from build123d import *

# Parameters (mm, degrees)
SKETCH_1_R          = 17
EXTRUDE_1_DEPTH     = 2
EXTRUDE_2_DEPTH     = 1
FILLET_1_R          = 1.55
FILLET_2_R          = 0.8
SKETCH_3_R          = 7
CUT_EXTRUDE_1_DEPTH = 4
SKETCH_4_R          = 1.25
CUT_EXTRUDE_2_DEPTH = 4.0000001


with BuildPart() as part:
    # ｽｹｯﾁ1 → ﾎﾞｽ - 押し出し1 (new body)
    with BuildSketch(Plane.XY):
        Circle(SKETCH_1_R)
    extrude(amount=EXTRUDE_1_DEPTH)

    # ｽｹｯﾁ2 → ﾎﾞｽ - 押し出し2 (add)
    with BuildSketch(Plane.XY.offset(2)):
        with BuildLine():
            Line((-1.5, 14.422205102), (-1.5, 12.5))
            Line((-1.5, 12.5), (1.5, 12.5))
            Line((1.5, 12.5), (1.5, 14.422205102))
            ThreePointArc((1.5, 14.422205102), (0, 14.5), (-1.5, 14.422205102))
        make_face()
        with BuildLine():
            Line((1.5, 12.5), (-1.5, 12.5))
            Line((-1.5, 12.5), (-1.5, 14.422205102))
            ThreePointArc((-1.5, 14.422205102), (-9.708243919, -10.770329614), (14.5, 0))
            ThreePointArc((14.5, 0), (10.770329614, 9.708243919), (1.5, 14.422205102))
            Line((1.5, 14.422205102), (1.5, 12.5))
        make_face()
        with BuildLine():
            Line((-1.5, 16.5), (-1.5, 14.422205102))
            ThreePointArc((-1.5, 14.422205102), (0, 14.5), (1.5, 14.422205102))
            Line((1.5, 14.422205102), (1.5, 16.5))
            Line((1.5, 16.5), (-1.5, 16.5))
        make_face()
    extrude(amount=EXTRUDE_2_DEPTH)

    # ﾌｨﾚｯﾄ1
    fillet_1_edges = [part.edges().sort_by_distance(p)[0] for p in [
        (-1.5, 14.422205102, 2.5),
        (1.5, 14.422205102, 2.5),
    ]]
    fillet(fillet_1_edges, radius=FILLET_1_R)

    # ﾌｨﾚｯﾄ2
    fillet_2_edges = [part.edges().sort_by_distance(p)[0] for p in [
        (1.5, 16.5, 2.5),
        (-1.5, 16.5, 2.5),
    ]]
    fillet(fillet_2_edges, radius=FILLET_2_R)

    # ｽｹｯﾁ3 → ｶｯﾄ - 押し出し1 (cut, through all)
    with BuildSketch(Plane.XY.offset(3)):
        Circle(SKETCH_3_R)
    extrude(amount=-CUT_EXTRUDE_1_DEPTH, mode=Mode.SUBTRACT)

    # ｽｹｯﾁ4 → ｶｯﾄ - 押し出し2 (cut, through all)
    with BuildSketch(Plane(origin=(0, 0, 0), x_dir=(-1, 0, 0), z_dir=(0, 0, -1))):
        with Locations((0, 12)):
            Circle(SKETCH_4_R)
        with Locations((12, 0)):
            Circle(SKETCH_4_R)
        with Locations((0, -12)):
            Circle(SKETCH_4_R)
        with Locations((-12, 0)):
            Circle(SKETCH_4_R)
    extrude(amount=-CUT_EXTRUDE_2_DEPTH, mode=Mode.SUBTRACT)


solid = part.part
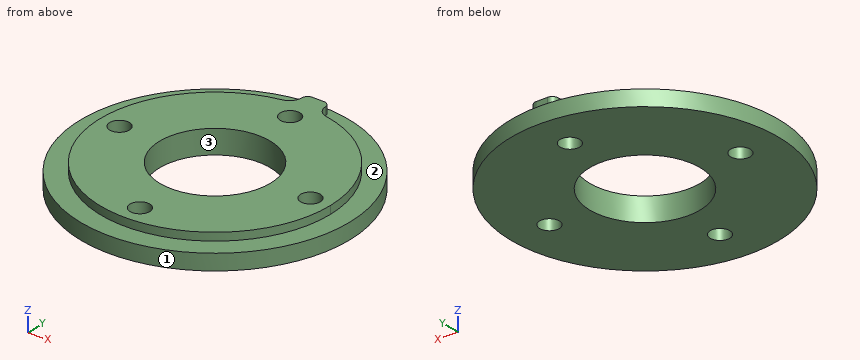
Input: part model. Units: mm. Frame: model coordinates. Face numbers are marked on the shaded views. Coordinates: 2 decimals unless noted, no trailing zeros. Loops run counter-clockwise (first coordinate to the right, second up) from the corner with the lowest first, then second, coordinate; pieces in that order, holes last.
Q1. Cut plane C-C (z = 0.65). Output: boundary loops of the cut face in (x, y), then the cut area to 3 significant figures.
Q2. Material intervals for line 1 (Y direction, x = 0, z = 1.5); line 2 (X direction, y = -1, z = 1.95); line 3 (Y direction, x = 11, z = 1.45), sorted ascending.
Q3. Draft query along Y for the marked faces 1, 2 and 3. Return one class per face: +Y half, -Y half, draft (parallel to the pull), parting line (faces both ways), or undercut.
Q4. Cut plane A-A (x = 0). Output: boundary loops of the cut face in (y, z).
Q5. Cut plane B-B (y = 12). Output: boundary loops of the cut face in (x, z).
Q6. Contact query for flat-ended pins moving along their axis: pin 1 (1.1 mm diameter, centred on x = 0, z = 2.5, fed in from +Y); pin 2 (1 mm diameter, centred on y = 12, z = 0.5, fed in from -X); pin 3 (1.5 mm diameter, centred on x = 12, z = 1.5, fed in from +Y). Output: stop coordinate, or through.
Working result:
1. outline: circle Ø34 at (0, 0); hole circle Ø2.5 at (-12, 0); hole circle Ø14 at (0, 0); hole circle Ø2.5 at (0, -12); hole circle Ø2.5 at (0, 12); hole circle Ø2.5 at (12, 0)
1. area: 734 mm2
2. line 1: y = -17 to -13.25, -10.75 to -7, 7 to 10.75, 13.25 to 17
2. line 2: x = -16.97 to -12.75, -11.25 to -6.93, 6.93 to 11.25, 12.75 to 16.97
2. line 3: y = -12.96 to -0.75, 0.75 to 12.96
3. face 1: parting line
3. face 2: draft
3. face 3: undercut
4. outline: (-17, 0) - (-13.25, 0) - (-13.25, 3) - (-14.5, 3) - (-14.5, 2) - (-17, 2) - close; (-10.75, 0) - (-7, 0) - (-7, 3) - (-10.75, 3) - close; (7, 0) - (10.75, 0) - (10.75, 3) - (7, 3) - close; (13.25, 0) - (17, 0) - (17, 2) - (16.5, 2) - (16.5, 3) - (13.25, 3) - close
5. outline: (-12.04, 0) - (-1.25, 0) - (-1.25, 3) - (-8.14, 3) - (-8.14, 2) - (-12.04, 2) - close; (1.25, 0) - (12.04, 0) - (12.04, 2) - (8.14, 2) - (8.14, 3) - (1.25, 3) - close
6. pin 1: stops at y = 17
6. pin 2: stops at x = -12.52
6. pin 3: stops at y = 12.75
